```python
from build123d import *

# Parameters (mm, degrees)
SKETCH4_R           = 14.5
SKETCH4_R_2         = 1.75
SKETCH4_R_3         = 4.5
BOSS_EXTRUDE5_DEPTH = 4
CUT_EXTRUDE1_DEPTH  = 2
CHAMFER1_SIZE       = 0.5


with BuildPart() as part:
    # Sketch4 → Boss-Extrude5 (new body)
    with BuildSketch(Plane.XY):
        Circle(SKETCH4_R)
        with Locations((0, 11.25)):
            Circle(SKETCH4_R_2, mode=Mode.SUBTRACT)
        with Locations((9.742785793, -5.625)):
            Circle(SKETCH4_R_2, mode=Mode.SUBTRACT)
        with Locations((-9.742785793, -5.625)):
            Circle(SKETCH4_R_2, mode=Mode.SUBTRACT)
        Circle(SKETCH4_R_3, mode=Mode.SUBTRACT)
    extrude(amount=BOSS_EXTRUDE5_DEPTH)

    # Sketch5 → Cut-Extrude1 (cut)
    with BuildSketch(Plane.XY.offset(4)):
        Polygon((12.742785793, -3.892949192), (9.742785793, -2.160898385), (6.742785793, -3.892949192), (6.742785793, -7.357050808), (9.742785793, -9.089101615), (11.4748366, -10.089101615), (14.4748366, -4.892949192), align=None)
        Polygon((-3, 12.982050808), (-3, 9.517949192), (0, 7.785898385), (3, 9.517949192), (3, 12.982050808), (3, 14.982050808), (-3, 14.982050808), align=None)
        Polygon((-9.742785793, -9.089101615), (-6.742785793, -7.357050808), (-6.742785793, -3.892949192), (-9.742785793, -2.160898385), (-12.742785793, -3.892949192), (-14.4748366, -4.892949192), (-11.4748366, -10.089101615), align=None)
    extrude(amount=-CUT_EXTRUDE1_DEPTH, mode=Mode.SUBTRACT)

    # Chamfer1
    chamfer1_edges = [part.edges().sort_by_distance(p)[0] for p in [
        (-11.492785793, -5.625, 0),
        (-4.5, 0, 0),
        (-4.5, 0, 4),
        (-14.5, 0, 0),
        (-12.557368355, 7.25, 4),
        (3, 11.852105076, 4),
        (-3, 11.852105076, 4),
        (-1.5, 8.651923789, 4),
        (1.5, 8.651923789, 4),
        (11.263880326, 9.130991184, 4),
        (-1.75, 11.25, 0),
        (8.764224084, -8.524128749, 4),
        (11.764224084, -3.327976327, 4),
        (8.242785793, -3.026923789, 4),
        (6.742785793, -5.625, 4),
        (0, -14.5, 4),
        (-11.764224084, -3.327976327, 4),
        (-8.764224084, -8.524128749, 4),
        (-6.742785793, -5.625, 4),
        (-8.242785793, -3.026923789, 4),
        (7.992785793, -5.625, 0),
    ]]
    chamfer(chamfer1_edges, length=CHAMFER1_SIZE)


solid = part.part
```
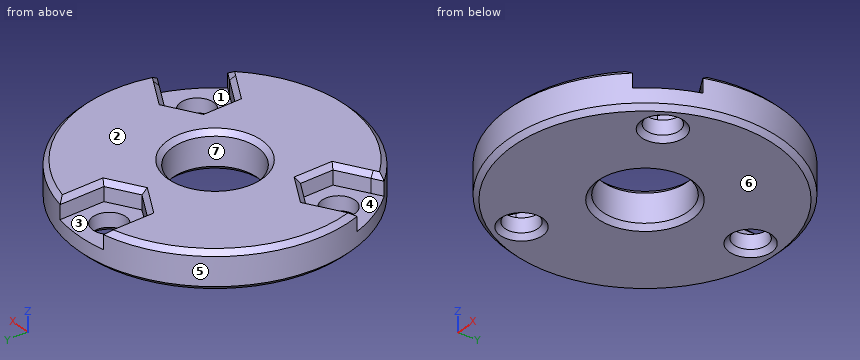
Work out the finished part from the listing and answer in its coordinate system (mm). Face numbers are marked on the shaded views. A direction names the side the tool comes from. Coordinates: 2 decimals unless noted, no trailing zeros. Loops run counter-clockwise (first coordinate to the right, second up) from the corner with the lowest first, then second, coordinate; pieces in that order, holes last.
1) For the marked faces 1, 2 and 3, determine the directions among +Z, -Z, +X, -X, +Y, -Y from which every point of the face is accessible in a straight line to the end or side of a thin tool.
Results:
face 1: +Z
face 2: +Z, +X, -X, +Y, -Y
face 3: +Z, +Y
2) Section A-A (y = 0) is taken. Give the vertices of the cut face in (x, z), plus the area to 3 significant figures.
Results:
outline: (-14.5, 0.5) - (-14, 0) - (-5, 0) - (-4.5, 0.5) - (-4.5, 3.5) - (-5, 4) - (-14, 4) - (-14.5, 3.5) - close; (4.5, 0.5) - (5, 0) - (14, 0) - (14.5, 0.5) - (14.5, 3.5) - (14, 4) - (5, 4) - (4.5, 3.5) - close
area: 79.0 mm2
3) Flat-ended cylindrical pins translate along their axes: pin 1 (1.5 mm diameter, centred on x = 10.5, z = 1.5, fed in from +Y); pin 2 (0.8 mm diameter, centred on y = -6, z = 3, fed in from -X); pin 3 (3 mm diameter, centred on x = -9.74, y = -5.62, fed in from +Z); pin 4 (0.8 mm diameter, centred on y = 11, z = 2.5, fed in from -X). Find the tip coordinate at first contact, or state that the pin passes through.
Results:
pin 1: stops at y = 10.73
pin 2: stops at x = -6.74
pin 3: passes through
pin 4: stops at x = -9.89
4) For a pull along X with two mould halves and no side action, classify the marked faces 4, 5, 6 and 7 as +X half, -X half, draft (parallel to the pull), parting line (faces both ways), or undercut.
Results:
face 4: undercut
face 5: parting line
face 6: draft
face 7: undercut
5) Consider probe 1 along Y at (x, z) = (1, 1.4); probe 2 along X at (y, z) = (-2.25, 3.65); probe 3 along X at (y, z) = (-6.5, 1.4). Determine where each line is inside the solid, lowest interval first.
Results:
probe 1: y = -14.47 to -4.39, 4.39 to 9.81, 12.69 to 14.47
probe 2: x = -14.17 to -10.2, -9.29 to -4.07, 4.07 to 9.29, 10.2 to 14.17
probe 3: x = -12.96 to -11.26, -8.23 to 8.23, 11.26 to 12.96
